from build123d import *
from build123d.topology import SkipClean

# Parameters (mm, degrees)
BOSS_EXTRUDE1_DEPTH = 6
BOSS_EXTRUDE4_START = 6
BOSS_EXTRUDE4_DEPTH = 6
CUT_EXTRUDE1_DEPTH  = 8
BOSS_EXTRUDE5_START = -12
SKETCH9_W           = 14.823924706
SKETCH9_H           = 3
BOSS_EXTRUDE5_DEPTH = 12
CUT_EXTRUDE3_DEPTH  = 10
CUT_EXTRUDE4_DEPTH  = 17.015617378
SKETCH12_W          = 7
SKETCH12_H          = 6
BOSS_EXTRUDE6_DEPTH = 2
SKETCH13_R          = 1
CUT_EXTRUDE5_DEPTH  = 18.344461472


with BuildPart() as part:
    # Sketch3 → Boss-Extrude1 (new body)
    with BuildSketch(Plane(origin=(0, 0, 0), x_dir=(1, 0, 0), z_dir=(0, 1, 0))):
        with BuildLine():
            Line((-6.25, 4.145780988), (6.25, 4.145780988))
            ThreePointArc((6.25, 4.145780988), (0, -7.5), (-6.25, 4.145780988))
        make_face()
    extrude(amount=BOSS_EXTRUDE1_DEPTH)

    # Sketch7 → Boss-Extrude4 (add)
    with SkipClean():  # the faces are left unmerged after this step: merging them gives an invalid solid
        with BuildSketch(Plane.XZ.offset(BOSS_EXTRUDE4_START)):
            with BuildLine():
                Line((6.25, -4.145780988), (-6.25, -4.145780988))
                ThreePointArc((-6.25, -4.145780988), (-6.993733183, -2.708818223), (-7.411962353, -1.145780988))
                Line((-7.411962353, -1.145780988), (7.411962353, -1.145780988))
                ThreePointArc((7.411962353, -1.145780988), (6.993733183, -2.708818223), (6.25, -4.145780988))
            make_face()
        extrude(amount=-BOSS_EXTRUDE4_DEPTH)

    # Sketch4 → Cut-Extrude1 (cut)
    with SkipClean():  # the faces are left unmerged after this step: merging them gives an invalid solid
        with BuildSketch(Plane(origin=(0, 6, 0), x_dir=(1, 0, 0), z_dir=(0, 1, 0))):
            with BuildLine():
                Line((-1.2489996, -0.854219012), (1.2489996, -0.854219012))
                ThreePointArc((1.2489996, -0.854219012), (0, -3.454219012), (-1.2489996, -0.854219012))
            make_face()
        extrude(amount=-CUT_EXTRUDE1_DEPTH, mode=Mode.SUBTRACT)

    # Sketch9 → Boss-Extrude5 (add)
    with BuildSketch(Plane.XZ.offset(6).offset(BOSS_EXTRUDE5_START)):
        with Locations((0, -2.645780988)):
            Rectangle(SKETCH9_W, SKETCH9_H)
    extrude(amount=BOSS_EXTRUDE5_DEPTH)

    # Sketch8 → Cut-Extrude3 (cut)
    with BuildSketch(Plane.XY.offset(-1.145780988)):
        with BuildLine():
            Line((-3, -2), (3, -2))
            ThreePointArc((3, -2), (4, -3), (3, -4))
            Line((3, -4), (-3, -4))
            ThreePointArc((-3, -4), (-4, -3), (-3, -2))
        make_face()
    extrude(amount=-CUT_EXTRUDE3_DEPTH, mode=Mode.SUBTRACT)

    # Sketch11 → Cut-Extrude4 (cut, through all)
    with BuildSketch(Plane(origin=(0, 6, 0), x_dir=(1, 0, 0), z_dir=(0, 1, 0))):
        with BuildLine():
            Line((-1, -7.433034374), (-1, -3.103218612))
            ThreePointArc((-1, -3.103218612), (0, -3.454219012), (1, -3.103218612))
            Line((1, -3.103218612), (1, -7.433034374))
            ThreePointArc((1, -7.433034374), (0, -7.5), (-1, -7.433034374))
        make_face()
    extrude(amount=-CUT_EXTRUDE4_DEPTH, mode=Mode.SUBTRACT)

    # Sketch12 → Boss-Extrude6 (add)
    with BuildSketch(Plane(origin=(-1, 0, 0), x_dir=(0, 0, -1), z_dir=(1, 0, 0))):
        with Locations((-8.933034374, 3)):
            Rectangle(SKETCH12_W, SKETCH12_H)
    boss_extrude6 = extrude(amount=-BOSS_EXTRUDE6_DEPTH)

    # Mirror1: Boss-Extrude6 across plane
    add(boss_extrude6.mirror(Plane(origin=(0, 0, 0), x_dir=(0, 0, 1), z_dir=(1, 0, 0))))

    # Sketch13 → Cut-Extrude5 (cut, through all)
    with BuildSketch(Plane.ZY.offset(3)):
        with Locations((9.653448958, 3)):
            Circle(SKETCH13_R)
    extrude(amount=-CUT_EXTRUDE5_DEPTH, mode=Mode.SUBTRACT)


solid = part.part
Could you check a few things on this model? Use its own coordinates, in mm. A direction names the side the tool comes from. Coordinates: 2 decimals unless noted, no trailing zeros. Order: outer loops, then holes, each group sorted by start corner. A loop starts at its lowest first (then second) coordinate and runs counter-clockwise, first axis right, second up. Notation, with made-up numbers: (24, -2.75) -> (72, -2.75) arc R7 ccw to (72, 9.25) -> close; hole circle Ø1 at (88, -29). An arc over 180 degrees is marked (long way). One line per question, with ' | ' between items.
Q1. Imagine slicing it at B-B on z = 7.75. Please give me the cut outline in (x, y).
Return value:
outline: (-3, 0) -> (-1, 0) -> (-1, 6) -> (-3, 6) -> close; (1, 0) -> (3, 0) -> (3, 6) -> (1, 6) -> close
Q2. If I drill on L1, parallel to X at y = 5.5, z = 7.25; L2, parallel to X at y = 5.5, z = -2.75; L3, parallel to Y at x = 6.5, z = 2, over which ranges is the centre line in solid material (lowest first)?
Return value:
L1: -3 to -1, 1 to 3 | L2: -7.41 to 7.41 | L3: 0 to 6
Q3. Imagine slicing it at C-C on y = 3. Please give me the cut outline in (x, z).
Return value:
outline: (-7.41, -4.15) -> (7.41, -4.15) -> (7.41, -1.15) arc R7.5 ccw to (3, 6.87) -> (3, 8.65) -> (1, 8.65) -> (1, 3.1) arc R1.6 cw to (1.25, 0.85) -> (-1.25, 0.85) arc R1.6 cw to (-1, 3.1) -> (-1, 8.65) -> (-3, 8.65) -> (-3, 6.87) arc R7.5 ccw to (-7.41, -1.15) -> close; (-3, 10.65) -> (-1, 10.65) -> (-1, 12.43) -> (-3, 12.43) -> close; (1, 10.65) -> (3, 10.65) -> (3, 12.43) -> (1, 12.43) -> close
Q4. Imagine slicing it at A-A on x = 2.25. Please give me the cut outline in (y, z), and give its area (3 significant figures).
Return value:
outline: (-6, -4.15) -> (-4, -4.15) -> (-4, -1.15) -> (-6, -1.15) -> close; (-2, -4.15) -> (6, -4.15) -> (6, 12.43) -> (0, 12.43) -> (0, -1.15) -> (-2, -1.15) -> close; hole circle Ø2 at (3, 9.65) | area: 108 mm²
Q5. Thinking about a two-plate mould opening in X: for faces 6 (the face through (-2, 3, 12.433)), 7 (the face through (6.604, 2.958, 3.555)), 8 (the face through (1, 3, 8)), which applies, pulls with the +X half, pulls with the -X half, needs draft (parallel to the pull), parting line crosses it, or undercut?
Return value:
face 6: needs draft | face 7: pulls with the +X half | face 8: undercut
Q6. On a 3-axis mill with a long thin cutter (end or side, diameter ignored), from which of +Z, -Z, +X, -X, +Y, -Y can I reach the whole of each face in a straight line? I mean faces 1 (the face through (3, 3, 11)), 2 (the face through (-1.588, 3.042, 2.048)), 3 (the face through (0, -2, -3)), 4 (the face through (-2, 0, 4)), 5 (the face through (7.412, 0, -3)). Say none if no direction works.
Return value:
face 1: +Z, +X, +Y, -Y | face 2: +Y, -Y | face 3: +Z, -Z | face 4: +Z, +X, -X, -Y | face 5: -Z, +X, +Y, -Y
Q7. I'm going to push flat-ended pins straight in: P1, Ø3.5, axis at y = -2, z = -2.5, coming from the +X side; P2, Ø1, axis at y = 3, z = 3, coming from the +X side; P3, Ø7, axis at x = 3.5, z = 9, coming from the -Y side; P4, Ø2.5, axis at x = 0.5, y = 1.5, coming from the +Z side. Where does each tip first touch, or does it pass through?
Return value:
P1: x = 7.41 | P2: x = 7.07 | P3: y = 0 | P4: z = 12.43
Q8. Imagine slicing it at D-D on z = -2. Please give me the cut outline in (x, y).
Return value:
outline: (-7.41, -6) -> (7.41, -6) -> (7.41, 6) -> (-7.41, 6) -> close; hole (-3, -4) -> (3, -4) arc R1 ccw to (3, -2) -> (-3, -2) arc R1 ccw to start
